```python
from build123d import *

# Parameters (mm, degrees)
COVER_BASE_DEPTH       = 27.5
SKIZZE2_W              = 25
SKIZZE2_H              = 18
CAMERA_COVER_CUT_DEPTH = 148.947625868
SKIZZE3_R              = 1.5
SPACER_SCREW_DEPTH     = 1
KREISMUSTER1_COUNT     = 4


with BuildPart() as part:
    # Skizze1 → Cover Base (new body)
    with BuildSketch(Plane.XY):
        with BuildLine():
            Line((69.309090313, 19.5), (53.5, 19.5))
            Line((53.5, 19.5), (53.5, 0))
            Line((53.5, 0), (54, 0))
            Line((54, 0), (54, 19))
            Line((54, 19), (69.966063202, 19))
            ThreePointArc((69.966063202, 19), (-9.584112318, 71.863723749), (-72.5, 0))
            Line((-72.5, 0), (-72, 0))
            ThreePointArc((-72, 0), (-9.842395478, 71.324100073), (69.309090313, 19.5))
        make_face()
    cover_base = extrude(amount=COVER_BASE_DEPTH)

    # Skizze2 → Camera Cover Cut (cut, through all)
    with BuildSketch(Plane(origin=(53.5, 0, 0), x_dir=(0, 0, -1), z_dir=(1, 0, 0))):
        with Locations((-15, 9)):
            Rectangle(SKIZZE2_W, SKIZZE2_H)
    camera_cover_cut = extrude(amount=CAMERA_COVER_CUT_DEPTH, mode=Mode.SUBTRACT)

    # Cover Mirror: Cover Base, Camera Cover Cut across plane
    add(cover_base.mirror(Plane.ZX))
    add(camera_cover_cut.mirror(Plane.ZX), mode=Mode.SUBTRACT)

    # Skizze3 → Spacer Screw (add)
    with BuildSketch(Plane.XY):
        with BuildLine():
            ThreePointArc((52.648755544, 49.113221638), (50.911688245, 50.911688245), (49.113221638, 52.648755544))
            Line((49.113221638, 52.648755544), (45.961940777, 49.497474683))
            ThreePointArc((45.961940777, 49.497474683), (45.961940777, 45.961940777), (49.497474683, 45.961940777))
            Line((49.497474683, 45.961940777), (52.648755544, 49.113221638))
        make_face()
        with Locations((47.72970773, 47.72970773)):
            Circle(SKIZZE3_R, mode=Mode.SUBTRACT)
    spacer_screw = extrude(amount=SPACER_SCREW_DEPTH)

    # Kreismuster1: Spacer Screw ×4 about axis
    kreismuster1_axis = Axis((0, 0, 0), (0, 0, 1))
    for i in range(1, KREISMUSTER1_COUNT):
        add(spacer_screw.rotate(kreismuster1_axis, i * 360 / KREISMUSTER1_COUNT))


solid = part.part
```
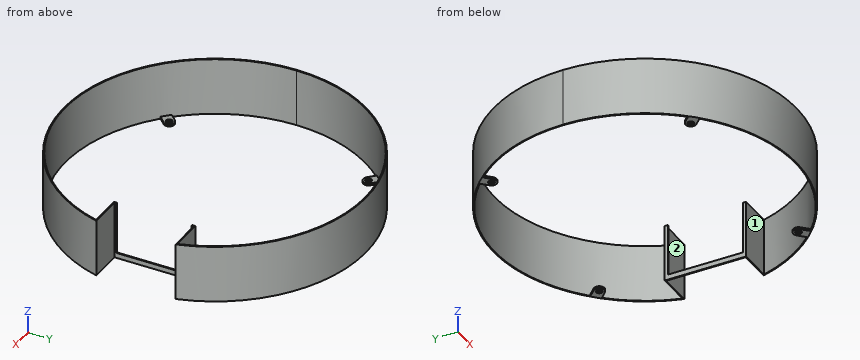
Geometry: final body of the model. Coordinates: model frame, mm. Face numbers are marked on the shaded views. Give positions to 0.01 mm unless a question says otherwise; leave off trailing zeros. Loops run counter-clockwise (first coordinate to the right, second up) from the corner with the lowest first, then second, coordinate; pieces in that order, holes last. Notation, with made-up numbers: (67.25, 33) -> (120.25, 33) arc R14 cw to (120.25, 42) -> close; hole circle Ø4 at (46.25, 50). An arc over 180 degrees is marked (long way). Return JSON: item names as keys, results as strings.
Item 1: Pin query (flat end, axial travel): P1, Ø4, axis at y = 35.5, z = 23, coming from the -X side; P2, Ø1.5, axis at x = -11.5, z = 3.5, coming from the +Y side; P3, Ø0.6, axis at x = 53.5, y = 3.5, coming from the +Z side; P4, Ø8, axis at y = 2, z = 13.5, coming from the -X side. Return the tip coordinate at first contact, or that it passes through.
Filled in:
{"P1": "x = -64.3", "P2": "y = 71.7", "P3": "z = 2.5", "P4": "x = -72.5"}
Item 2: Section B-B, the plane x = -14.5. Output: boundary loops of the cut face in (y, z).
Filled in:
{"outline": "(-71.04, 0) -> (-70.52, 0) -> (-70.52, 27.5) -> (-71.04, 27.5) -> close; (70.52, 0) -> (71.04, 0) -> (71.04, 27.5) -> (70.52, 27.5) -> close"}
Item 3: Section D-D, the plane x = 61.5. Output: boundary loops of the cut face in (y, z).
Filled in:
{"outline": "(-38.39, 0) -> (-37.44, 0) -> (-37.44, 27.5) -> (-38.39, 27.5) -> close; (-19.5, 0) -> (-19, 0) -> (-19, 27.5) -> (-19.5, 27.5) -> close; (19, 0) -> (19.5, 0) -> (19.5, 27.5) -> (19, 27.5) -> close; (37.44, 0) -> (38.39, 0) -> (38.39, 27.5) -> (37.44, 27.5) -> close"}
Item 4: Mould query, pull axis X, two halves, no side actions, for the marked faces 1 and 2. Classes: released by +X, released by -X, zero draft, split by the parting line, or undercut.
Filled in:
{"face 1": "undercut", "face 2": "zero draft"}
Item 5: Line query: line 1 (Y direction, x = -2, z = 14.5); line 2 (Y direction, x = 47, z = 8.5); line 3 (X direction, y = -59.5, z = 1.75). Output: solid intervals per line, ascending.
Filled in:
{"line 1": "-72.47 to -71.97, 71.97 to 72.47", "line 2": "-55.2 to -54.54, 54.54 to 55.2", "line 3": "-41.42 to -40.54, 40.54 to 41.42"}
Item 6: Section C-C, the plane z = 5.5. Output: boundary loops of the cut face in (x, y), plus the area to 3 significant figures.
Filled in:
{"outline": "(53.5, -19.5) -> (69.31, -19.5) arc R72 cw (long way) to (69.31, 19.5) -> (53.5, 19.5) -> (53.5, 18) -> (54, 18) -> (54, 19) -> (69.97, 19) arc R72.5 ccw (long way) to (69.97, -19) -> (54, -19) -> (54, -18) -> (53.5, -18) -> close", "area": "225 mm^2"}
